```python
from build123d import *

# Parameters (mm, degrees)
SKETCH_1_R               = 6
EXTRUDE_1_DEPTH          = 45
SKETCH_2_R               = 7.5
EXTRUDE_2_DEPTH          = 12.7
SKETCH_3_R               = 6
EXTRUDE_3_DEPTH          = 20
SKETCH_4_R               = 5
EXTRUDE_4_DEPTH          = 5
SKETCH_5_R               = 4
EXTRUDE_5_DEPTH          = 7.3
SKETCH_6_R               = 3
EXTRUDE_6_DEPTH          = 12
CUT_EXTRUDE_1_DEPTH      = 103.549987811
CUT_EXTRUDE_1_DEPTH_BACK = 103.549987811
SKETCH_7_R               = 2.1
CUT_EXTRUDE_2_DEPTH      = 103.549987811
CUT_EXTRUDE_2_DEPTH_BACK = 103.549987811
SKETCH_8_R               = 1.65


with BuildPart() as part:
    # ｽｹｯﾁ1 → ﾎﾞｽ - 押し出し1 (new body)
    with BuildSketch(Plane(origin=(0, 0, 0), x_dir=(0, 0, -1), z_dir=(1, 0, 0))):
        with Locations(Location((0, 0, 0), (0, 0, 180))):
            Circle(SKETCH_1_R)
    extrude(amount=EXTRUDE_1_DEPTH)

    # ｽｹｯﾁ2 → ﾎﾞｽ - 押し出し2 (add)
    with BuildSketch(Plane(origin=(45, 0, 0), x_dir=(0, 0, -1), z_dir=(1, 0, 0))):
        Circle(SKETCH_2_R)
    extrude(amount=EXTRUDE_2_DEPTH)

    # ｽｹｯﾁ3 → ﾎﾞｽ - 押し出し3 (add)
    with BuildSketch(Plane(origin=(57.7, 0, 0), x_dir=(0, 0, -1), z_dir=(1, 0, 0))):
        with Locations(Location((0, 0, 0), (0, 0, 180))):
            Circle(SKETCH_3_R)
    extrude(amount=EXTRUDE_3_DEPTH)

    # ｽｹｯﾁ4 → ﾎﾞｽ - 押し出し4 (add)
    with BuildSketch(Plane(origin=(77.7, 0, 0), x_dir=(0, 0, -1), z_dir=(1, 0, 0))):
        Circle(SKETCH_4_R)
    extrude(amount=EXTRUDE_4_DEPTH)

    # ｽｹｯﾁ5 → ﾎﾞｽ - 押し出し5 (add)
    with BuildSketch(Plane(origin=(82.7, 0, 0), x_dir=(0, 0, -1), z_dir=(1, 0, 0))):
        Circle(SKETCH_5_R)
    extrude(amount=EXTRUDE_5_DEPTH)

    # ｽｹｯﾁ6 → ﾎﾞｽ - 押し出し6 (add)
    with BuildSketch(Plane(origin=(90, 0, 0), x_dir=(0, 0, -1), z_dir=(1, 0, 0))):
        Circle(SKETCH_6_R)
    extrude(amount=EXTRUDE_6_DEPTH)

    # ｽｹｯﾁ7 → ｶｯﾄ - 押し出し1 (cut, two sides: drawn at the far end of the back side and taken through both)
    with BuildSketch(Plane(origin=(0, 0, 0), x_dir=(1, 0, 0), z_dir=(0, 1, 0)).offset(-CUT_EXTRUDE_1_DEPTH_BACK)):
        with Locations(Location((25, 0, 0), (0, 0, 270))):
            Circle(SKETCH_7_R)
        with Locations(Location((5, 0, 0), (0, 0, 270))):
            Circle(SKETCH_7_R)
    extrude(amount=CUT_EXTRUDE_1_DEPTH + CUT_EXTRUDE_1_DEPTH_BACK, mode=Mode.SUBTRACT)

    # ｽｹｯﾁ8 → ｶｯﾄ - 押し出し2 (cut, two sides: drawn at the far end of the back side and taken through both)
    with BuildSketch(Plane(origin=(0, 0, 0), x_dir=(1, 0, 0), z_dir=(0, 1, 0)).offset(-CUT_EXTRUDE_2_DEPTH_BACK)):
        with Locations(Location((62.7, 0, 0), (0, 0, 270))):
            Circle(SKETCH_8_R)
    extrude(amount=CUT_EXTRUDE_2_DEPTH + CUT_EXTRUDE_2_DEPTH_BACK, mode=Mode.SUBTRACT)


solid = part.part
```
Build history of the part. All positions in model axes, mm. A direction names the side the tool comes from. Round coordinates to 2 decimals unless told otherwise and drop trailing zeros. Write each loop counter-clockwise with the first axis right and the second up, starting at its lowest first coordinate (ties: lowest second). Pieces come first, ordered by that corner, then holes.
1) 3-axis set-ups, long thin cutter, end or side, ignore diameter. For faces 4 (the flat face through (102, 0, 0)), 5 (the flat face through (45, 6, -2)), 6 (the cylindrical face through (96, 0, 3)): which of +Z, -Z, +X, -X, +Y, -Y reach the whole face in a straight line?
2) Band-saw the part on C-C, the plane x = 62.7. List the corners of the cut face in (y, z).
3) Band-saw the part on A-A, the plane z = 0. Give the number of separate pieces and of enclosed holes in the cut face, and give its area (3 significant figures).
4) Band-saw the part on D-D, the plane x = 86.5. List the corners of the cut face in (y, z).
5) Band-saw the part on B-B, the plane x = 14. List the corners of the cut face in (y, z).
6) Drill centre lines: probe 1 along X at (y, z) = (3.25, 0); probe 2 along X at (y, z) = (2, 0); probe 3 along Z at (x, y) = (62.7, -0.25). Where is each one in solid material? Low to high.
7) Pin check, flat tips, straight feed: pin 1 (5 mm diameter, centred on x = 87, y = -4, fed in from +Z); pin 2 (3 mm diameter, centred on y = -3, z = -4, fed in from +X); pin 3 (1 mm diameter, centred on x = 84, z = 0, fed in from +Y). Stop position of each tip, or through.
8) Mould opens along Z. For faces 1 (the cylindrical face through (22.185, -1.802, 5.723)), 2 (the flat face through (90, 3, -1)), 3 (the cylindrical face through (7.082, -0.084, -0.273)) say: +Z half, -Z half, draft (parallel to the pull), parting line (faces both ways), or undercut.
Ans:
1. face 4: +Z, -Z, +X, +Y, -Y
1. face 5: -X
1. face 6: +X
2. outline: (-5.77, -1.65) arc R6 ccw to (5.77, -1.65) - close; (-5.77, 1.65) - (5.77, 1.65) arc R6 ccw to start
3. separate pieces: 4
3. enclosed holes: 0
3. area: 1,010 mm2
4. outline: circle Ø8 at (0, 0)
5. outline: circle Ø12 at (0, 0)
6. probe 1: x = 0 to 2.9, 7.1 to 22.9, 27.1 to 61.05, 64.35 to 90
6. probe 2: x = 0 to 2.9, 7.1 to 22.9, 27.1 to 61.05, 64.35 to 102
6. probe 3: z = -5.99 to -1.65, 1.65 to 5.99
7. pin 1: stops at z = 3.71
7. pin 2: stops at x = 90
7. pin 3: stops at y = 4
8. face 1: parting line
8. face 2: draft
8. face 3: undercut
